Geometry check sheet. Reference: the model listing, model coordinates, mm. Coordinates: 2 decimals unless noted, no trailing zeros. Write each loop counter-clockwise with the first axis right and the second up, starting at its lowest first coordinate (ties: lowest second). Pieces come first, ordered by that corner, then holes.
from build123d import *

# Parameters (mm, degrees)
F1_DEPTH = 2.54


with BuildPart() as f1:
    # F0 (on Top) → F1 (new body)
    with BuildSketch(Plane.XY):
        with BuildLine():
            Line((99.615625, 0), (0, 0))
            Line((0, 0), (0, -163.195))
            Line((0, -163.195), (25.4, -163.195))
            ThreePointArc((25.4, -163.195), (26.213694, -161.230569), (28.178125, -160.416875))
            Line((28.178125, -160.416875), (55.165625, -160.416875))
            ThreePointArc((55.165625, -160.416875), (55.863077, -158.733077), (57.546875, -158.035625))
            Line((57.546875, -158.035625), (59.928125, -158.035625))
            ThreePointArc((59.928125, -158.035625), (61.611923, -158.733077), (62.309375, -160.416875))
            Line((62.309375, -160.416875), (78.58125, -160.416875))
            ThreePointArc((78.58125, -160.416875), (80.545681, -161.230569), (81.359375, -163.195))
            Line((81.359375, -163.195), (83.740625, -163.195))
            Line((83.740625, -163.195), (91.678125, -8.89))
            Line((91.678125, -8.89), (99.615625, -1.27))
            Line((99.615625, -1.27), (99.615625, 0))
        make_face()
    extrude(amount=F1_DEPTH)


solid = f1.part
1. Sectioned sample at B-B, the plane x = 38.5. Record the boundary of the cut face in (y, z), and give its area (3 significant figures).
Computed values:
outline: (-160.42, 0) - (0, 0) - (0, 2.54) - (-160.42, 2.54) - close
area: 407 mm2
2. Thickness scan on line 1 along Y through (x, z) = (64.5, 0.5); line 2 along Y through (x, z) = (59, 0.8); line 3 along X through (y, z) = (-128, 0.85). Record the ranges inside material, lowest first.
Computed values:
line 1: y = -160.42 to 0
line 2: y = -158.04 to 0
line 3: x = 0 to 85.55
3. Sectioned sample at A-A, the plane z = 0.6. Record the boundary of the cut face in (x, y) (1 decimal).
Computed values:
outline: (0, -163.2) - (25.4, -163.2) arc R2.8 cw to (28.2, -160.4) - (55.2, -160.4) arc R2.4 cw to (57.5, -158) - (59.9, -158) arc R2.4 cw to (62.3, -160.4) - (78.6, -160.4) arc R2.8 cw to (81.4, -163.2) - (83.7, -163.2) - (91.7, -8.9) - (99.6, -1.3) - (99.6, 0) - (0, 0) - close
4. Sectioned sample at C-C, the plane y = -116.5. Record the boundary of the cut face in (x, z), and give its area (3 significant figures).
Computed values:
outline: (0, 0) - (86.14, 0) - (86.14, 2.54) - (0, 2.54) - close
area: 219 mm2
5. Draft check along Y on faces 1 (the flat face through (49, -80, 0)), 2 (the flat face through (95.591, -5.133, 1.252)). Enter one of: released by +Y, released by -Y, zero draft, split by the parting line, or undercut.
Computed values:
face 1: zero draft
face 2: released by -Y
6. Gauge pin test, flat ends, axial feed: pin 1 Ø1 at (x, z) = (56.5, 0.5) entering from -Y; pin 2 Ø2 at (x, y) = (53.5, -43) entering from -Z; pin 3 Ø1.2 at (x, z) = (59, 1.5) entering from -Y. Record the tip position at first contact, or that the pin passes through.
Computed values:
pin 1: stops at y = -158.61
pin 2: stops at z = 0
pin 3: stops at y = -158.04
